Source: CAD feature listing. Evaluate the final solid. Frame: model axes, mm. Face numbers are marked on the shaded views. A direction names the side the tool comes from. Give positions to 0.01 mm unless a question says otherwise; leave off trailing zeros. Loops run counter-clockwise (first coordinate to the right, second up) from the corner with the lowest first, then second, coordinate; pieces in that order, holes last. Notation, with made-up numbers: M 33.25,58 L 81.25,58 A15 ccw 81.25,87 Z; hole C 16.25,67.5 d1. An arc over 180 degrees is marked long. Put each result on its own line as item: value.
from build123d import *

# Parameters (mm, degrees)
SKETCH_W        = 170
SKETCH_H        = 135
PAD_DEPTH       = 3
SKETCH001_W     = 26
SKETCH001_H     = 135
PAD001_DEPTH    = 90
SKETCH004_W     = 20
SKETCH004_H     = 136.715439
POCKET_DEPTH    = 90
SKETCH006_W     = 20
SKETCH006_H     = 57.5
PAD002_DEPTH    = 60
SKETCH007_W     = 17.5
SKETCH007_H     = 54.5
POCKET001_DEPTH = 60
SKETCH008_R     = 25
PAD003_DEPTH    = 6
SKETCH009_R     = 23
POCKET002_DEPTH = 6


with BuildPart() as part:
    # Sketch → Pad (new body)
    with BuildSketch(Plane.XY):
        Rectangle(SKETCH_W, SKETCH_H)
    extrude(amount=PAD_DEPTH)

    # Sketch001 (on Face6 of Pad) → Pad001 (join)
    with BuildSketch(Plane.XY.offset(3)):
        with Locations((72, 0)):
            Rectangle(SKETCH001_W, SKETCH001_H)
    extrude(amount=PAD001_DEPTH)

    # Sketch004 (on Face10 of Pad001) → Pocket (cut)
    with BuildSketch(Plane.XY.offset(93)):
        with Locations((71.988623, -3.85772)):
            Rectangle(SKETCH004_W, SKETCH004_H)
    extrude(amount=-POCKET_DEPTH, mode=Mode.SUBTRACT)

    # Sketch006 (on Face5 of Pocket) → Pad002 (join)
    with BuildSketch(Plane.XY.offset(3)):
        with Locations((49, -38.75)):
            Rectangle(SKETCH006_W, SKETCH006_H)
    extrude(amount=PAD002_DEPTH)

    # Sketch007 (on Face17 of Pad002) → Pocket001 (cut)
    with BuildSketch(Plane.XY.offset(63)):
        with Locations((50.223179, -40.25)):
            Rectangle(SKETCH007_W, SKETCH007_H)
    extrude(amount=-POCKET001_DEPTH, mode=Mode.SUBTRACT)

    # Sketch008 (on Face5 of Pocket001) → Pad003 (join)
    with BuildSketch(Plane.XY.offset(3)):
        with Locations((-59.057144, -41.630726)):
            Circle(SKETCH008_R)
    extrude(amount=PAD003_DEPTH)

    # Sketch009 (on Face21 of Pad003) → Pocket002 (cut)
    with BuildSketch(Plane.XY.offset(9)):
        with Locations((-59.057144, -41.630726)):
            Circle(SKETCH009_R)
    extrude(amount=-POCKET002_DEPTH, mode=Mode.SUBTRACT)


solid = part.part
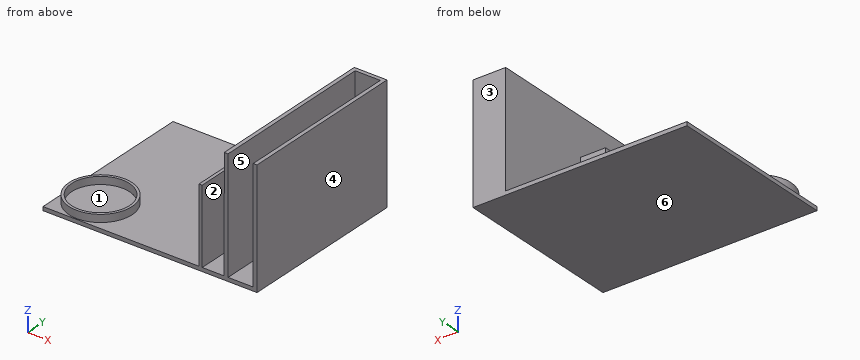
1. Draft query along X for the marked faces 4, 5 and 6. Return one class per face: pulls with the +X half, pulls with the -X half, needs draft (parallel to the pull), parting line crosses it, or undercut.
Found:
face 4: pulls with the +X half
face 5: undercut
face 6: needs draft
2. Section query B-B (x = 47.5). Output: boundary loops of the cut face in (y, z).
Found:
outline: M -67.5,0 L 67.5,0 L 67.5,3 L -10,3 L -10,63 L -13,63 L -13,3 L -67.5,3 Z
3. Material intervals for line 1 (X direction, y = -34, z = 48); line 2 (X direction, y = -29, z = 87); line 3 (Z direction, x = -49.5, y = 48), sorted ascending. Write a range as from..to.
Found:
line 1: 39..41.47, 58.97..61.99, 81.99..85
line 2: 59..61.99, 81.99..85
line 3: 0..3
4. Section query A-A (z = 85). Output: boundary loops of the cut face in (x, y), plus the area to 3 significant figures.
Found:
outline: M 59,-67.5 L 61.99,-67.5 L 61.99,64.5 L 81.99,64.5 L 81.99,-67.5 L 85,-67.5 L 85,67.5 L 59,67.5 Z
area: 870 mm^2
5. Access query for the marked faces 1, 2 and 3. Directions: +Z, -Z, +X, -X, +Y, -Y. A direction counts if a zero-diameter tool reaches every point of the face in a straight line with its end or side. Return the directions, or none.
Found:
face 1: +Z
face 2: +Z, -Y
face 3: +Z, -Z, +X, -X, +Y
6. Section query D-D (z = 17.5). Output: boundary loops of the cut face in (x, y).
Found:
outline: M 39,-67.5 L 41.47,-67.5 L 41.47,-13 L 58.97,-13 L 58.97,-67.5 L 61.99,-67.5 L 61.99,64.5 L 81.99,64.5 L 81.99,-67.5 L 85,-67.5 L 85,67.5 L 59,67.5 L 59,-10 L 39,-10 Z
7. Contact query for flat-ended pins moving along their axis: P1, Ø16, axis at x = 72, y = -19.5, coming from the +Z side; P2, Ø16, axis at x = 73.5, z = 69, coming from the -Y side; P3, Ø16, axis at x = 47.5, z = 32.5, coming from the +Y side; P4, Ø1, axis at x = 54.5, z = 65, coming from the -Y side. Output: stop coordinate, or through.
Found:
P1: z = 3
P2: y = 64.5
P3: y = -10
P4: through
